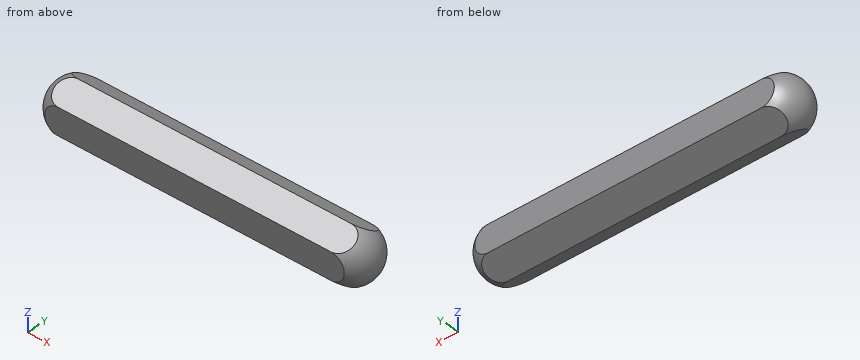
```python
from build123d import *

# Parameters (mm, degrees)
OCTAGONAL_CUT_DEPTH      = 27.280030441382678
OCTAGONAL_CUT_DEPTH_BACK = 27.280030441382678


with BuildPart() as part:
    # Sketch1 → Body Revolve (revolve)
    with BuildSketch(Plane.XY):
        with BuildLine():
            Line((-21.400000000000002, 4.2), (21.400000000000002, 4.200000000000008))
            ThreePointArc((21.400000000000002, 4.200000000000008), (24.3698484809835, 2.9698484809835084), (25.6, 9.41e-15))
            Line((25.6, 9.41e-15), (-25.6, 0))
            ThreePointArc((-25.6, 0), (-24.369848480983503, 2.9698484809835), (-21.400000000000002, 4.2))
        make_face()
    revolve(axis=Axis((-25.6, 0, 0), (1, 1.8e-16, 0)))

    # Sketch2 → Octagonal Cut (cut, two sides: drawn at the far end of the back side and taken through both)
    with BuildSketch(Plane(origin=(0, 0, 0), x_dir=(0, 0, -1), z_dir=(1, 0, 0)).offset(-OCTAGONAL_CUT_DEPTH_BACK)):
        with BuildLine():
            Line((-4.1999999999999975, 8.44e-15), (-2.0999999999999983, 3.637306695894651))
            ThreePointArc((-2.099999999999999, 3.637306695894651), (-3.6373066958946416, 2.10000000000001), (-4.2, 9.15e-15))
        make_face()
        with BuildLine():
            ThreePointArc((2.1000000000000005, 3.6373066958946505), (2.6e-16, 4.200000000000009), (-2.099999999999999, 3.637306695894651))
            Line((-2.0999999999999983, 3.637306695894651), (2.1, 3.6373066958946496))
        make_face()
        with BuildLine():
            ThreePointArc((4.2, 8.63e-15), (3.6373066958946425, 2.100000000000008), (2.1000000000000005, 3.6373066958946505))
            Line((2.1, 3.6373066958946496), (4.199999999999999, 8.08e-15))
        make_face()
        with BuildLine():
            ThreePointArc((2.1000000000000005, -3.6373066958946336), (3.6373066958946434, -2.0999999999999903), (4.2, 7.61e-15))
            Line((4.199999999999999, 7.99e-15), (2.1, -3.6373066958946327))
        make_face()
        with BuildLine():
            Line((2.1000000000000005, -3.6373066958946327), (-2.0999999999999988, -3.637306695894634))
            ThreePointArc((-2.0999999999999983, -3.637306695894635), (-7.7e-16, -4.199999999999991), (2.1000000000000005, -3.6373066958946336))
        make_face()
        with BuildLine():
            Line((-2.0999999999999988, -3.637306695894634), (-4.1999999999999975, 8.2e-15))
            ThreePointArc((-4.2, 9.15e-15), (-3.637306695894642, -2.099999999999992), (-2.0999999999999983, -3.637306695894635))
        make_face()
    extrude(amount=OCTAGONAL_CUT_DEPTH + OCTAGONAL_CUT_DEPTH_BACK, mode=Mode.SUBTRACT)


solid = part.part
```
Part model, mm, in its own coordinate system. Round coordinates to 2 decimals unless told otherwise and drop trailing zeros. Write each loop counter-clockwise with the first axis right and the second up, starting at its lowest first coordinate (ties: lowest second). Pieces come first, ordered by that corner, then holes. Notation, with made-up numbers: (23, 47.5) -> (82, 47.5) arc R16 ccw to (82, 63.5) -> close; hole circle Ø6 at (14, 14.5). An arc over 180 degrees is marked (long way). Return JSON: item names as keys, results as strings. Group by question number.
Q1. Saw through at C-C on z = 1. Write the cut outline in (x, y).
Q2. Pin check, flat tip, straight feed: pin 1 (3 mm diameter, centred on x = 1, y = -2.5, fed in from +Z). Stop position of the tip, or through.
Q3. Saw through at B-B on y = -1. Write the cut outline in (x, z).
Q4. Saw through at A-A on x = 12.5. Write the cut outline in (y, z), plus the area to 3 significant figures.
Q5. Probe L1, parallel to X at y = -0.25, z = 2.5; L2, parallel to Z at x = 14, y = 0.25; L3, parallel to Y at x = -14, z = -3.25. List the from-to ranges inside material, lowest first. Write a range as [from, to].
Answer:
{
 "1": {"outline": "(-23.25, -3.64) -> (23.25, -3.64) arc R4.08 ccw to (23.25, 3.64) -> (-23.25, 3.64) arc R4.08 ccw to start"},
 "2": {"pin 1": "z = 3.62"},
 "3": {"outline": "(-23.28, -3.62) -> (23.28, -3.62) arc R4.08 ccw to (23.28, 3.62) -> (-23.28, 3.62) arc R4.08 ccw to start"},
 "4": {"outline": "(-3.64, -2.1) -> (0, -4.2) -> (3.64, -2.1) -> (3.64, 2.1) -> (0, 4.2) -> (-3.64, 2.1) -> close", "area": "45.8 mm2"},
 "5": {"L1": "[-24.77, 24.77]", "L2": "[-4.06, 4.06]", "L3": "[-1.65, 1.65]"}
}
